Verification items for this drawing (mm, ordinates from the low corner). A direction names the side the tool comes from. Round coordinates to 2 decimals unless told otherwise and drop trailing zeros. Order: outer loops, then holes, each group sorted by start corner. A loop starts at its lowest first (then second) coordinate and runs counter-clockwise, first axis right, second up. Notation, with made-up numbers: (11, 54.5) -> (18, 54.5) arc R26 ccw to (18, 72.5) -> close; hole circle Ø1 at (19.5, -36.75). An arc over 180 degrees is marked (long way). Use a Markdown table: item, result. Add a question column.
Item 1: Set-up check for the marked faces 1, 2 and 3: record each of +Z, -Z, +X, -X, +Y, -Y from which the full face is reachable in a straight line by a thin tool's end or side.
Item 2: Material ranges on probe 1 along X at (y, z) = (69.85, 44.25); probe 2 along Z at (x, y) = (29, 16.5); probe 3 along Y at (x, z) = (38.1, 49.25) (1 decimal), recorded low to high. Write a range as [from, to].
Item 3: Gauge pin test, flat ends, axial feed: pin 1 Ø19 at (x, y) = (41, 54) entering from -Z; pin 2 Ø1 at (y, z) = (31.5, 39.5) entering from -X; pin 3 Ø2.5 at (x, y) = (38.1, 69.85) entering from +Z; pin 4 Ø19 at (y, z) = (23, 42.5) entering from +X. Record the tip position at first contact, or that the pin passes through.
Item 4: Sectioned sample at C-C, the plane y = 60. Record the cut outline in (x, z).
Item 5: Sectioned sample at B-B, the plane x = 38.1. State how many separate pieces and enclosed holes the cut face has, and give its area (3 significant figures).
Item 6: Sectioned sample at A-A, the plane y = 69.85. Record the cut outline in (x, z), and give its area (3 significant figures).
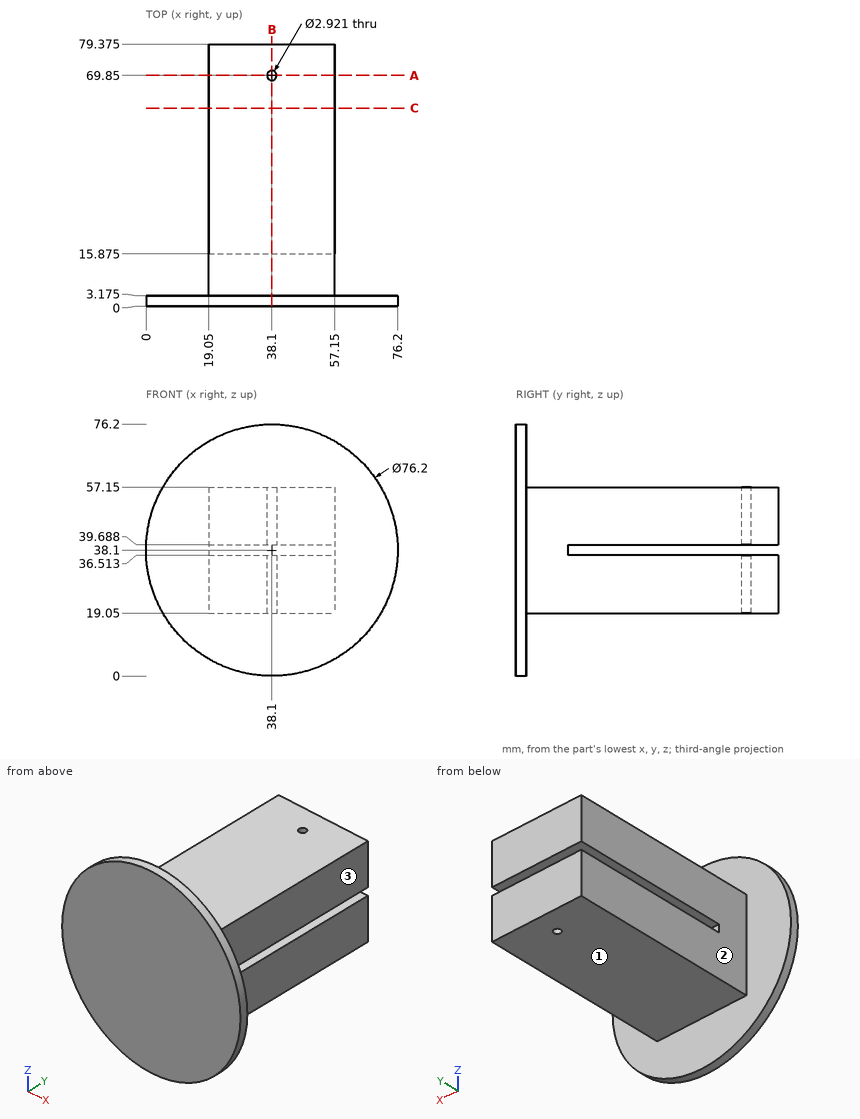
Found:
| question | item | result |
|---|---|---|
| 1 | face 1 | -Z, +X, -X, +Y |
| 1 | face 2 | +Z, -Z, -X, +Y |
| 1 | face 3 | +Z, -Z, +X, +Y |
| 2 | probe 1 | x = [19.05, 36.64], [39.56, 57.15] |
| 2 | probe 2 | z = [19.05, 36.51], [39.69, 57.15] |
| 2 | probe 3 | y = [0, 68.4], [71.3, 79.4] |
| 3 | pin 1 | stops at z = 19.05 |
| 3 | pin 2 | stops at x = 19.05 |
| 3 | pin 3 | passes through |
| 3 | pin 4 | stops at x = 57.15 |
| 4 | outline | (19.05, 19.05) -> (57.15, 19.05) -> (57.15, 36.51) -> (19.05, 36.51) -> close; (19.05, 39.69) -> (57.15, 39.69) -> (57.15, 57.15) -> (19.05, 57.15) -> close |
| 5 | separate pieces | 3 |
| 5 | enclosed holes | 0 |
| 5 | area | 2,840 mm2 |
| 6 | outline | (19.05, 19.05) -> (36.64, 19.05) -> (36.64, 36.51) -> (19.05, 36.51) -> close; (19.05, 39.69) -> (36.64, 39.69) -> (36.64, 57.15) -> (19.05, 57.15) -> close; (39.56, 19.05) -> (57.15, 19.05) -> (57.15, 36.51) -> (39.56, 36.51) -> close; (39.56, 39.69) -> (57.15, 39.69) -> (57.15, 57.15) -> (39.56, 57.15) -> close |
| 6 | area | 1,230 mm2 |
